CAD build for the part. Positions are in the model's coordinates, mm. Face numbers are marked on the shaded views. Give positions to 0.01 mm unless a question says otherwise; leave off trailing zeros. Loops run counter-clockwise (first coordinate to the right, second up) from the corner with the lowest first, then second, coordinate; pieces in that order, holes last. Notation, with made-up numbers: (-29.5, 53.5) -> (21.5, 53.5) arc R21 ccw to (21.5, 83.5) -> close; hole circle Ø9 at (-35, 11). An arc over 180 degrees is marked (long way). Use one line per item in the form item = value.
```python
from build123d import *

# Parameters (mm, degrees)
F0_W          = 60
F0_H          = 60
F1_DEPTH      = 25
F1_DEPTH_BACK = 25
F3_R          = 14.685213
F4_DEPTH      = 60.001
F5_R          = 10
F6_SIZE2      = 5
F6_SIZE       = 5


with BuildPart() as f1:
    # F0 (on Top) → F1 (new body, two sides)
    with BuildSketch(Plane.XY) as f1_sk:
        Rectangle(F0_W, F0_H)
    extrude(amount=F1_DEPTH)
    extrude(f1_sk.sketch, amount=-F1_DEPTH_BACK)

    # F3 (on offset) → F4 (cut, through all)
    with BuildSketch(Plane(origin=(-30, 0, 0), x_dir=(0, -1, 0), z_dir=(-1, 0, 0))):
        Circle(F3_R)
    extrude(amount=-F4_DEPTH, mode=Mode.SUBTRACT)

    # F5
    f5_edges = [f1.edges().sort_by_distance(p)[0] for p in [
        (0, 30, -25),
        (0, 30, 25),
        (0, -30, 25),
        (0, -30, -25),
    ]]
    fillet(f5_edges, radius=F5_R)

    # F6
    f6_edges = [f1.edges().sort_by_distance(p)[0] for p in [
        (30, 30, 0),
        (-30, 30, 0),
    ]]
    chamfer(f6_edges, length=F6_SIZE, length2=F6_SIZE2)


solid = f1.part
```
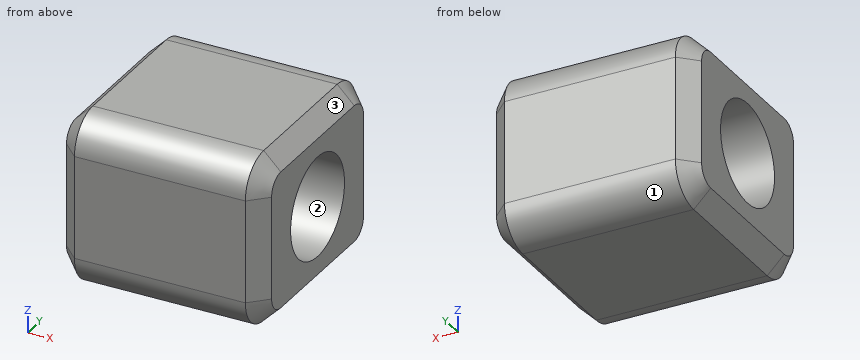
1. Drop a flat-ended pin along its axis: P1, Ø2, axis at x = 11.5, z = 19, coming from the -Y side. Give the stop position or say it passes through.
Result sheet:
P1 = -29.54
2. Cut at D-D, the plane y = -18. Write the cut outline in (x, z), then the cut area to 3 significant figures.
Result sheet:
outline = (-30, -20) -> (-25, -25) -> (25, -25) -> (30, -20) -> (30, 20) -> (25, 25) -> (-25, 25) -> (-30, 20) -> close
area = 2,950 mm^2
3. Mould opens along Y. For the marked faces 1, 2 and 3 say: pulls with the +Y half, pulls with the -Y half, needs draft (parallel to the pull), parting line crosses it, or undercut.
Result sheet:
face_1 = pulls with the +Y half
face_2 = undercut
face_3 = needs draft
4. Cut at C-C, the plane z = 0. Write the cut outline in (x, y).
Result sheet:
outline = (-30, -25) -> (-25, -30) -> (25, -30) -> (30, -25) -> (30, -14.69) -> (-30, -14.69) -> close; (-30, 14.69) -> (30, 14.69) -> (30, 25) -> (25, 30) -> (-25, 30) -> (-30, 25) -> close
5. Drill centre lines: line 1 (Z direction, x = -12, y = 0); line 2 (Y direction, x = 18, z = -13); line 3 (Y direction, x = 24.5, z = -12). Where is each one in solid material? Low to high.
Result sheet:
line_1 = -25 to -14.69, 14.69 to 25
line_2 = -30 to -6.83, 6.83 to 30
line_3 = -30 to -8.46, 8.46 to 30
6. Cut at A-A, the plane y = 0. Write the cut outline in (x, z).
Result sheet:
outline = (-30, -20) -> (-25, -25) -> (25, -25) -> (30, -20) -> (30, -14.69) -> (-30, -14.69) -> close; (-30, 14.69) -> (30, 14.69) -> (30, 20) -> (25, 25) -> (-25, 25) -> (-30, 20) -> close
7. Cut at B-B, the plane x = 21.5. Write the cut outline in (y, z), then the cut area to 3 significant figures.
Result sheet:
outline = (-30, -15) arc R10 ccw to (-20, -25) -> (20, -25) arc R10 ccw to (30, -15) -> (30, 15) arc R10 ccw to (20, 25) -> (-20, 25) arc R10 ccw to (-30, 15) -> close; hole circle Ø29.37 at (0, 0)
area = 2,240 mm^2
